Verification items for the finished model (mm, model axes). Face numbers are marked on the shaded views. A direction names the side the tool comes from. Coordinates: 2 decimals unless noted, no trailing zeros. Order: outer loops, then holes, each group sorted by start corner. A loop starts at its lowest first (then second) coordinate and runs counter-clockwise, first axis right, second up. Notation, with made-up numbers: (58, -36) -> (79, -36) arc R7 ccw to (79, -30) -> close; hole circle Ø7 at (80.25, 62). An arc over 180 degrees is marked (long way). Write item = value, one per line. Start each with the question number.
Autodesk Inventor part; units mm, degrees
ref_plane "YZ Plane" through (0, 0, 0) normal (1, 0, 0) x (0, 1, 0)
ref_plane "XZ Plane" through (0, 0, 0) normal (0, 1, 0) x (-1, 0, 0)
ref_plane "XY Plane" through (0, 0, 0) normal (0, 0, 1) x (1, 0, 0)
sketch "Sketch1" plane through (0, 0, 0) normal (0, 0, 1) x (1, 0, 0)
  line L0 (-7, 0) -> (7, 0)
  line L1 (0, -38.5) -> (0, 38.5)
  line L2 (5, 25) -> (5, -25)
  line L3 (-5, -25) -> (-5, 25)
  line L4 (-2.5, -25) -> (-2.5, -27.5)
  line L5 (-2.5, -27.5) -> (2.5, -27.5)
  line L6 (2.5, -27.5) -> (2.5, -25)
  line L7 (5, -25) -> (2.5, -25)
  line L8 (-2.5, -25) -> (-5, -25)
  line L9 (-2.5, 25) -> (-2.5, 27.5)
  line L10 (-2.5, 27.5) -> (2.5, 27.5)
  line L11 (2.5, 27.5) -> (2.5, 25)
  line L12 (-5, 25) -> (-2.5, 25)
  line L13 (2.5, 25) -> (5, 25)
  point P0 (0, 0)
  dimension "d0" = 10
  dimension "d1" = 50
  dimension "d3" = 5
  dimension "d7" = 2.5
  dimension "d8" = 2.5
  dimension "d10" = 2.5
  dimension "d11" = 2.5
  dimension "d12" = 2.5
extrude "Extrusion1" add sketch "Sketch1" along normal blind 2.2
equation "\"d3\" = 0.5 * d0"
equation "\"d2\" = 0.5 * d1"
properties part number "Acrylic_2.2_Lower"
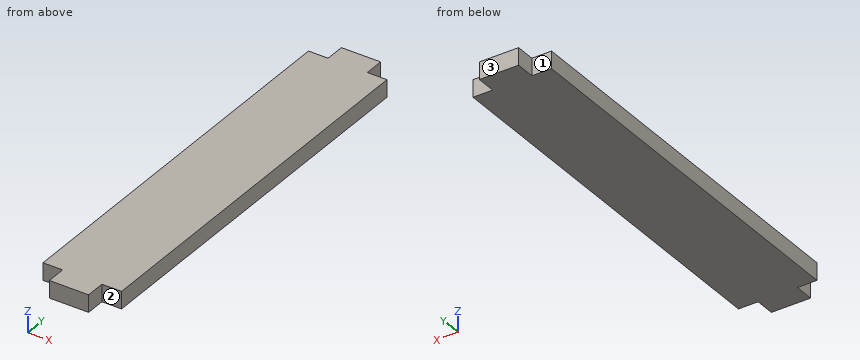
Item 1: Section check A-A (z = 1.65). Record the boundary of the cut face in (x, y), then the cut area to 3 significant figures.
Item 2: Thickness scan on line 1 (Y direction, x = 3.25, z = 2). Record the ranges inside material, lowest first.
Item 3: Gauge pin test, flat ends, axial feed: P1, Ø0.7, axis at x = 3.5, z = 1, coming from the -Y side; P2, Ø1.1, axis at y = 26, z = 1, coming from the -X side; P3, Ø1.1, axis at x = -4.5, z = 1, coming from the +Y side. Record the tip position at first contact, or that the pin passes through.
Item 4: Section check B-B (x = 3.25). Record the boundary of the cut face in (y, z).
Item 5: Tool access check on the marked faces 1, 2 and 3. Record the directions out of +Z, -Z, +X, -X, +Y, -Y that give a thin tool (end or side, any length) a straight path to the whole face; none if there is none.
Filled sheet:
q1.outline = (-5, -25) -> (-2.5, -25) -> (-2.5, -27.5) -> (2.5, -27.5) -> (2.5, -25) -> (5, -25) -> (5, 25) -> (2.5, 25) -> (2.5, 27.5) -> (-2.5, 27.5) -> (-2.5, 25) -> (-5, 25) -> close
q1.area = 525 mm^2
q2.line_1 = -25 to 25
q3.P1 = -25
q3.P2 = -2.5
q3.P3 = 25
q4.outline = (-25, 0) -> (25, 0) -> (25, 2.2) -> (-25, 2.2) -> close
q5.face_1 = +Z, -Z, -X, +Y
q5.face_2 = +Z, -Z, +X, -Y
q5.face_3 = +Z, -Z, +X, -X, +Y
